```python
from build123d import *

# Parameters (mm, degrees)
SKETCH_1_R          = 18.25
EXTRUDE_1_DEPTH     = 10
SKETCH_3_R          = 15
CUT_EXTRUDE_1_DEPTH = 8
SKETCH_4_R          = 20
SKETCH_4_R_2        = 15
EXTRUDE_2_DEPTH     = 70
SKETCH_5_R          = 20
SKETCH_5_R_2        = 18.5
EXTRUDE_3_DEPTH     = 10
FILLET_1_R          = 10


with BuildPart() as part:
    # 草图1 → 凸台-拉伸1 (new body)
    with BuildSketch(Plane(origin=(0, 0, 0), x_dir=(1, 0, 0), z_dir=(0, 1, 0))):
        with Locations(Location((0, 0, 0), (0, 0, 270))):
            Circle(SKETCH_1_R)
    extrude(amount=EXTRUDE_1_DEPTH)

    # 草图3 → 切除-拉伸1 (cut)
    with BuildSketch(Plane.XZ):
        with Locations(Location((0, 0, 0), (0, 0, 270))):
            Circle(SKETCH_3_R)
    extrude(amount=-CUT_EXTRUDE_1_DEPTH, mode=Mode.SUBTRACT)

    # 草图4 → 凸台-拉伸2 (add)
    with BuildSketch(Plane(origin=(0, 10, 0), x_dir=(1, 0, 0), z_dir=(0, 1, 0))):
        with Locations(Location((0, 0, 0), (0, 0, 270))):
            Circle(SKETCH_4_R)
        with Locations(Location((0, 0, 0), (0, 0, 90))):
            Circle(SKETCH_4_R_2, mode=Mode.SUBTRACT)
    extrude(amount=EXTRUDE_2_DEPTH)

    # 草图5 → 凸台-拉伸3 (add)
    with BuildSketch(Plane(origin=(0, 80, 0), x_dir=(1, 0, 0), z_dir=(0, 1, 0))):
        with Locations(Location((0, 0, 0), (0, 0, 270))):
            Circle(SKETCH_5_R)
        with Locations(Location((0, 0, 0), (0, 0, 270))):
            Circle(SKETCH_5_R_2, mode=Mode.SUBTRACT)
    extrude(amount=EXTRUDE_3_DEPTH)

    # 圆角1
    # the kernel refuses this fillet: 10 mm, written as the material it takes off along each edge
    with BuildSketch(Plane(origin=(0, 80, 0), x_dir=(0, 0, -1), z_dir=(1, 0, 0))) as fillet_1_piece_1:
        with BuildLine():
            CenterArc((25, -7.599342077), FILLET_1_R, 130.541601874, 49.458398126)
            Line((15, -7.599342077), (14.8, -7.599342077))
            Line((14.8, -7.599342077), (14.8, 0))
            Line((14.8, 0), (15, 0.2))
            ThreePointArc((15, 0.2), (16.75, 0.2), (18.37, 0.151986842))
            Line((18.37, 0.151986842), (18.5, 0))
        make_face()
    revolve(axis=Axis((0, 80, 0), (0, 1, 0)), mode=Mode.SUBTRACT)


solid = part.part
```
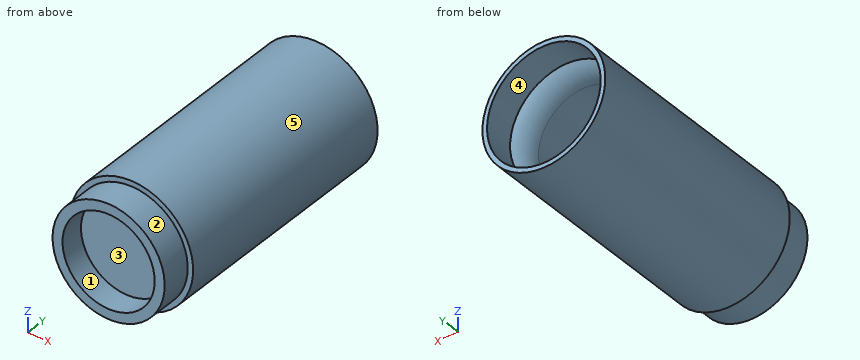
Design review of the part built by this model. Coordinates are the model's own, in mm. Face numbers are marked on the shaded views. A direction names the side the tool comes from. Coordinates: 2 decimals unless noted, no trailing zeros. Loops run counter-clockwise (first coordinate to the right, second up) from the corner with the lowest first, then second, coordinate; pieces in that order, holes last.
Q1. To check wall thickness, follow line 1 (X direction, y = 4, z = 0); line 2 (X direction, y = 25, z = 0); line 3 (Y direction, x = 8.5, z = 0.5). State the ranges of each line that lie inside material, in increasing order.
Reported:
line 1: x = -18.25 to -15, 15 to 18.25
line 2: x = -20 to -15, 15 to 20
line 3: y = 8 to 10
Q2. The part is to be moulded in two halves that separate along X. For the marked faces 1 and 2, say which applies: +X half, -X half, draft (parallel to the pull), parting line (faces both ways), or undercut.
Reported:
face 1: undercut
face 2: parting line
Q3. We need section B-B on y = 81. State the section outline as (x, z) points, and give its area (3 significant figures).
Reported:
outline: circle Ø40 at (0, 0); hole circle Ø37 at (0, 0)
area: 181 mm2
Q4. For pin 1 (8 mm diameter, centred on y = 60.5, z = 5.5, fed in from -X); pin 2 (10 mm diameter, centred on y = 78.5, z = -4.5, fed in from -X); pin 3 (1 mm diameter, centred on x = -9.5, y = 62, fed in from +Z), all flat-tipped, find the tip position at first contact; note any pin that passes through.
Reported:
pin 1: stops at x = -19.94
pin 2: stops at x = -20
pin 3: stops at z = 17.86
Q5. Tool access review of the marked faces 3, 4 and 5: name each direction out of +Z, -Z, +X, -X, +Y, -Y from which nothing blocks a thin tool from reaching the whole face with its end or side.
Reported:
face 3: -Y
face 4: +Y
face 5: +Y, -Y
Q6. We need section D-D on y = 56.5. State the section outline as (x, z) points, and give its area (3 significant figures).
Reported:
outline: circle Ø40 at (0, 0); hole circle Ø30 at (0, 0)
area: 550 mm2
Q7. We need section A-A on z = 0. State the section outline as (x, y) points.
Reported:
outline: (-20, 10) - (-18.25, 10) - (-18.25, 0) - (-15, 0) - (-15, 8) - (15, 8) - (15, 0) - (18.25, 0) - (18.25, 10) - (20, 10) - (20, 90) - (18.5, 90) - (18.5, 80) arc R10 ccw to (15, 72.4) - (15, 10) - (-15, 10) - (-15, 72.4) arc R10 ccw to (-18.5, 80) - (-18.5, 90) - (-20, 90) - close
Q8. We need section C-C on x = 0. State the section outline as (y, z) points.
Reported:
outline: (0, -18.25) - (10, -18.25) - (10, -20) - (90, -20) - (90, -18.5) - (80, -18.5) arc R10 ccw to (72.4, -15) - (10, -15) - (10, 15) - (72.4, 15) arc R10 ccw to (80, 18.5) - (90, 18.5) - (90, 20) - (10, 20) - (10, 18.25) - (0, 18.25) - (0, 15) - (8, 15) - (8, -15) - (0, -15) - close
